The figure shows three views and two pictorial views of one solid part (mm, origin at its lowest corner). Answer the questions. A direction names the side the tool comes from. Coordinates: 2 decimals unless noted, no trailing zeros. Write each loop counter-clockwise with the first axis right and the second up, starting at its lowest first coordinate (ties: lowest second). Pieces come first, ordered by that corner, then holes.
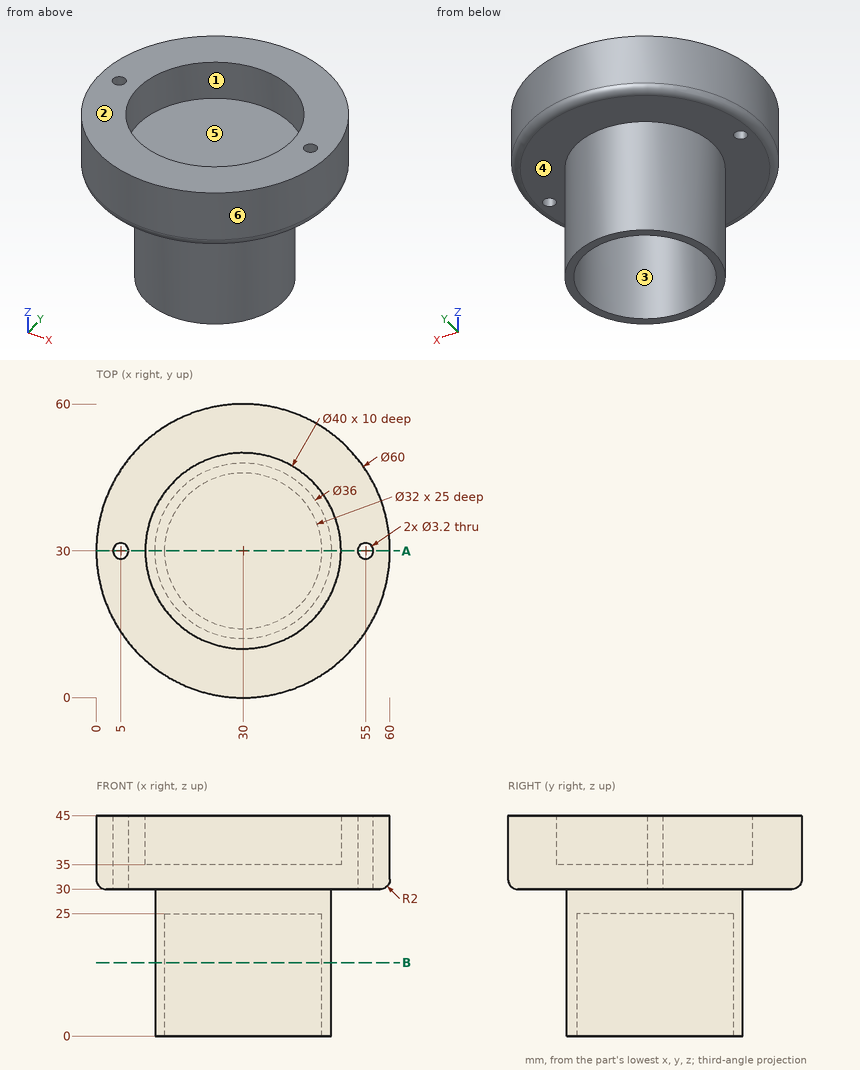
Q1. Find the intervals of material crossed by probe 1 along Y at (x, z) = (30, 17.5); probe 2 along Z at (x, y) = (12, 25); probe 3 along Y at (x, z) = (55, 41.5), in increasing order.
Answers below:
probe 1: y = 12 to 14, 46 to 48
probe 2: z = 30 to 35
probe 3: y = 13.42 to 28.4, 31.6 to 46.58
Q2. The part is cut by section A-A, the plane y = 30. Write down the section's boundary in (x, z), then the cut area to 3 significant figures.
Answers below:
outline: (0, 32) arc R2 ccw to (2, 30) - (3.4, 30) - (3.4, 45) - (0, 45) - close; (6.6, 30) - (12, 30) - (12, 0) - (14, 0) - (14, 25) - (46, 25) - (46, 0) - (48, 0) - (48, 30) - (53.4, 30) - (53.4, 45) - (50, 45) - (50, 35) - (10, 35) - (10, 45) - (6.6, 45) - close; (56.6, 30) - (58, 30) arc R2 ccw to (60, 32) - (60, 45) - (56.6, 45) - close
area: 682 mm2
Q3. Which of the six approach directions +Z, -Z, +X, -X, +Y, -Y give full straight-line access (tool end or side, diameter ignored) to the marked faces 1, 2 and 3?
Answers below:
face 1: +Z
face 2: +Z, +X, -X, +Y, -Y
face 3: -Z
Q4. Determine the mould class of the marked faces 4, 5 and 6 for opening direction Y: released by +Y, released by -Y, zero draft, split by the parting line, or undercut.
Answers below:
face 4: zero draft
face 5: undercut
face 6: split by the parting line
Q5. The part is cut by section B-B, the plane z = 15. Write down the section's boundary in (x, y).
Answers below:
outline: circle Ø36 at (30, 30); hole circle Ø32 at (30, 30)
Q6. Given pin 1 (3.5 mm diameter, centred on x = 5, y = 30, fed in from -Z); pin 2 (8 mm diameter, centred on y = 36.5, z = 11.5, fed in from -X); pin 3 (1.5 mm diameter, centred on x = 34.5, y = 25.5, fed in from +Z), each flat-ended and moving along its own axis, determine where each tip first touches the part or whether it passes through.
Answers below:
pin 1: stops at z = 30
pin 2: stops at x = 12.17
pin 3: stops at z = 35
